from build123d import *

# Parameters (mm, degrees)
F0_W   = 0.9
F0_H   = 6.62
F0_W_2 = 24.3
F0_H_2 = 4.305


with BuildPart() as f1:
    # F0 (on Right) → F1 (revolve)
    with BuildSketch(Plane.YZ):
        Polygon((0, 7.15), (0, 0), (0.5, 0), (1.52, 0), (1.52, 6.62), (1.52, 7.65), (0.5, 7.65), align=None)
        with Locations((1.97, 3.31)):
            Rectangle(F0_W, F0_H)
        Polygon((2.42, 6.62), (2.42, 0), (3.12, 0), (3.12, 7.455), align=None)
        Polygon((3.12, 7.455), (3.12, 0), (54.9, 0), (54.9, 6.91), align=None)
        Polygon((54.9, 6.91), (54.9, 0), (60.89, 0), (60.89, 4.73), align=None)
        Polygon((60.89, 4.73), (60.89, 0), (69.2, 0), (69.2, 4.305), (69.2, 4.705), align=None)
        with Locations((81.35, 2.1525)):
            Rectangle(F0_W_2, F0_H_2)
    revolve(axis=Axis((0, 29.01, 0), (0, 1, 0)))


solid = f1.part
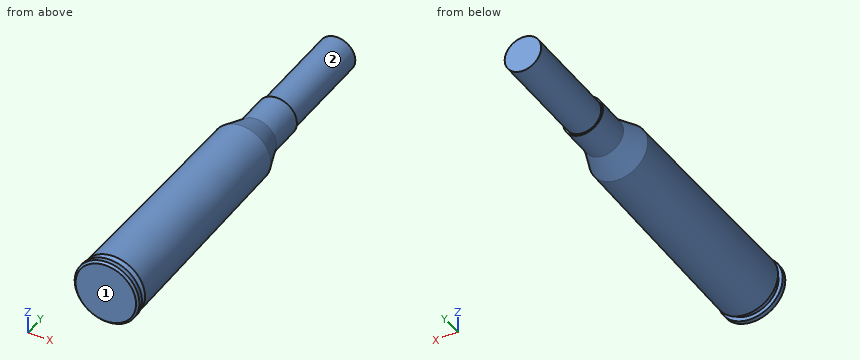
Build history of the part. All positions in model axes, mm. Face numbers are marked on the shaded views. A direction names the side the tool comes from. Round coordinates to 2 decimals unless told otherwise and drop trailing zeros. Write each loop counter-clockwise with the first axis right and the second up, starting at its lowest first coordinate (ties: lowest second). Pieces come first, ordered by that corner, then holes. Notation, with made-up numbers: (64, -22) -> (91, -22) arc R23 cw to (91, 17) -> close; hole circle Ø4 at (38.25, -18). An arc over 180 degrees is marked (long way). Write item = value, one per line.
(1) Band-saw the part on A-A (y = 82.5). Give the cut face in (x, z) (3 decimals), then the cut area to 3 significant figures.
Answer:
outline = circle Ø8.61 at (0, 0)
area = 58.2 mm2
(2) Band-saw the part on B-B (y = 50). Give the cut face in (x, z), then the cut area to 3 significant figures.
Answer:
outline = circle Ø13.92 at (0, 0)
area = 152 mm2
(3) Flat gauge pins, fed straight in: pin 1 (3 mm diameter, centred on y = 54, z = 4, fed in from +X); pin 2 (8 mm diameter, centred on y = 72, z = -0.5, fed in from -X); pin 3 (1 mm diameter, centred on x = -3.5, y = 39, fed in from +Z). Where does each tip first touch, or does it go through?
Answer:
pin_1 = 6.45
pin_2 = -4.71
pin_3 = 6.41
(4) Tool access for the marked faces 1 and 2: list every direction of +Z, -Z, +X, -X, +Y, -Y with a clear straight run to the whole face (end or side of a thin tool).
Answer:
face_1 = +Z, -Z, +X, -X, -Y
face_2 = +Y
(5) Probe L1, parallel to X at y = 39, z = 2.5; L2, parallel to Y at x = 4.25, z = 1.5; L3, parallel to Y at x = 3.25, z = 6.75. List the from-to ranges inside material, lowest first.
Answer:
L1 = -6.62 to 6.62
L2 = 0 to 69.2
L3 = 0.34 to 1.52
